Drawing for the job (mm, zero at the part's lowest x, y, z). A direction names the side the tool comes from. Coordinates: 2 decimals unless noted, no trailing zeros. Write each loop counter-clockwise with the first axis right and the second up, starting at its lowest first coordinate (ties: lowest second). Pieces come first, ordered by that corner, then holes. Notation, with made-up numbers: M -22,66 L 20,66 A24 ccw 20,91 Z; hole C -21.5,77 d1. An arc over 180 degrees is marked long. Use CSV: the item, a comma, the result in double quotes. Start each with the question number.
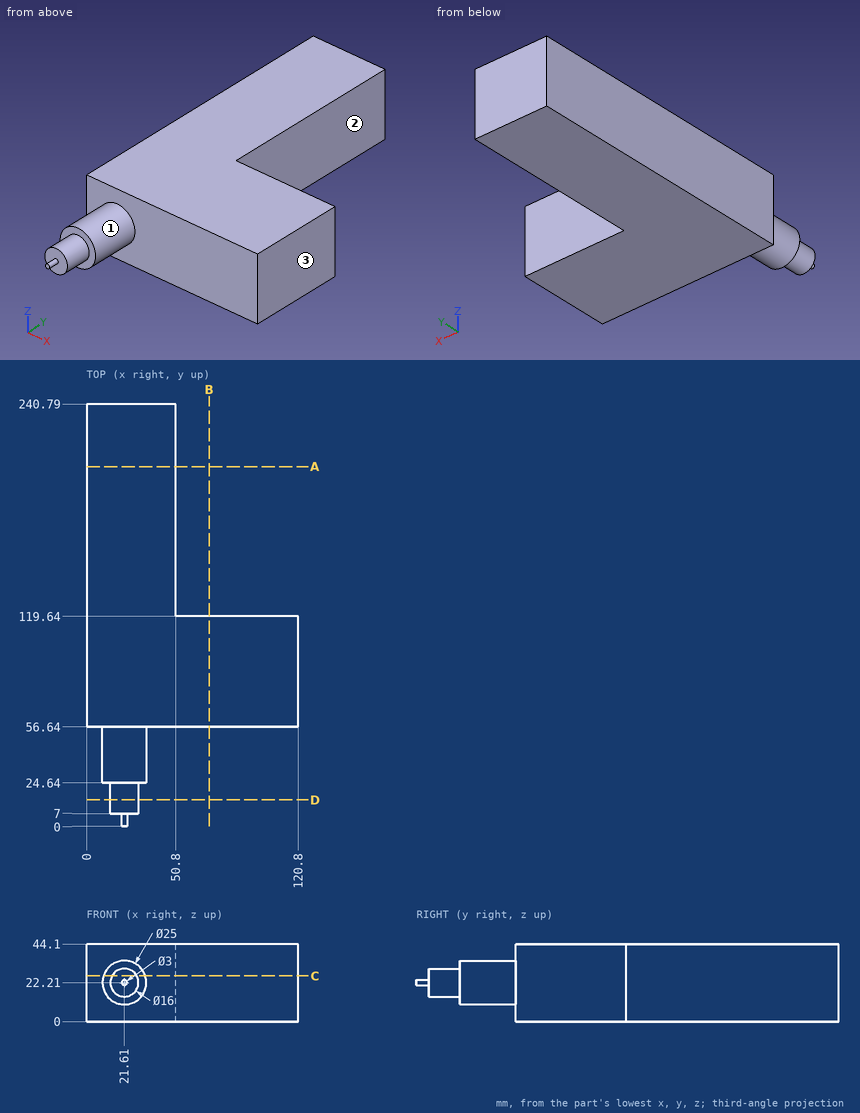
1) Wall check: L1, parallel to Y at x = 82.5, z = 31; L2, parallel to Y at x = 40, z = 13; L3, parallel to X at y = 154, z = 4. Give the ranges that are in metal, low to high. Write a range as [from, to].
2) Band-saw the part on C-C on z = 26. List the corners of the cut face in (x, y).
3) Band-saw the part on D-D on y = 15. List the corners of the cut face in (x, z), then the cut area to 3 significant figures.
4) Tool access for the marked faces 1, 2 and 3: list every direction of +Z, -Z, +X, -X, +Y, -Y with a clear straight run to the whole face (end or side of a thin tool).
5) Drop flat-ended pins along their axis: P1, Ø13, axis at x = 66.5, z = 19.5, coming from the -Y side; P2, Ø7.5, axis at x = 27, z = 21.5, coming from the -Y side; P3, Ø2, axis at y = 128.5, z = 16, coming from the +X side; P4, Ø3, axis at x = 80.5, y = 85.5, coming from the -Z side. Give the stop position or say it passes through.
6) Band-saw the part on A-A on y = 205. List the corners of the cut face in (x, z), then the cut area to 3 significant figures.
7) Band-saw the part on B-B on x = 70. List the corners of the cut face in (y, z), then the cut area to 3 significant figures.
Findings below:
1,L1,"y = [56.64, 119.64]"
1,L2,"y = [56.64, 240.79]"
1,L3,"x = [0, 50.8]"
2,outline,"M 0,56.64 L 9.7,56.64 L 9.7,24.64 L 14.56,24.64 L 14.56,7 L 28.66,7 L 28.66,24.64 L 33.52,24.64 L 33.52,56.64 L 120.8,56.64 L 120.8,119.64 L 50.8,119.64 L 50.8,240.79 L 0,240.79 Z"
3,outline,"C 21.61,22.21 d16"
3,area,"201 mm2"
4,face 1,"-Y"
4,face 2,"+Z, -Z, +X, +Y"
4,face 3,"+Z, -Z, +X, +Y, -Y"
5,P1,"stops at y = 56.64"
5,P2,"stops at y = 7"
5,P3,"stops at x = 50.8"
5,P4,"stops at z = 0"
6,outline,"M 0,0 L 50.8,0 L 50.8,44.1 L 0,44.1 Z"
6,area,"2,240 mm2"
7,outline,"M 56.64,0 L 119.64,0 L 119.64,44.1 L 56.64,44.1 Z"
7,area,"2,780 mm2"
